Autodesk Inventor part; units mm, degrees
ref_plane "YZ Plane" through (0, 0, 0) normal (1, 0, 0) x (0, 1, 0)
ref_plane "XZ Plane" through (0, 0, 0) normal (0, 1, 0) x (-1, 0, 0)
ref_plane "XY Plane" through (0, 0, 0) normal (0, 0, 1) x (1, 0, 0)
sketch "Sketch1" plane through (0, 0, 0) normal (0, 0, 1) x (1, 0, 0)
  circle A0 centre (0, 0) radius 2 construction
  circle A1 centre (0, 0) radius 6.5 construction
  line L0 (0, 0) -> (38, 0) construction
  arc A2 (-6.8763, 10.4387) -> (-6.8763, -10.4387) centre (0, 0) ccw
  circle A3 centre (0, 0) radius 6.5
  line L1 (38, 0) -> (38, -40)
  line L2 (38, 0) -> (38, 40)
  line L3 (38, 40) -> (-6.8763, 10.4387)
  line L4 (38, -40) -> (-6.8763, -10.4387)
  point P0 (0, 0)
  dimension "d0" = 38
  dimension "d1" = 25
  dimension "d2" = 13
  dimension "d3" = 40
  dimension "d4" = 40
extrude "Extrusion1" add sketch "Sketch1" against normal blind 6
sketch "Sketch2" plane through (0, 0, -6) normal (0, 0, -1) x (-1, 0, 0)
  circle A0 centre (-13, -12.5) radius 1.5
  circle A1 centre (-13, 12.5) radius 1.5
  point P0 (0, 0)
extrude "Extrusion2" cut sketch "Sketch2" against normal blind 6
sketch "Sketch3" plane through (0, 0, -6) normal (0, 0, -1) x (-1, 0, 0)
  line L0 (-38, 40) -> (-38, -40)
  line L1 (-38, 40) -> (-38, -40) construction
  line L2 (-38, 0) -> (-63, 0) construction
  line L3 (-50, 0) -> (-50, -17)
  line L4 (-50, 0) -> (-50, 17)
  line L5 (-50, -17) -> (-38, -17)
  line L6 (-50, 17) -> (-38, 17)
  line L7 (-47.1, -14) -> (-47.1, 0)
  line L8 (-47.1, 14) -> (-47.1, 0)
  line L9 (-47.1, -14) -> (-44, -14)
  line L10 (-44, -14) -> (-44, 0)
  line L11 (-47.1, 14) -> (-44, 14)
  line L12 (-44, 14) -> (-44, 0)
  line L13 (-38, -17) -> (-38, 17)
  point P0 (0, 0)
  dimension "d9" = 25
  dimension "d10" = 17
  dimension "d11" = 12
  dimension "d12" = 14
  dimension "d13" = 2.9
  dimension "d14" = 6
extrude "Extrusion3" add sketch "Sketch3" against normal blind 6
properties part number "Mecanum wheel support"
CAD build for the part. Positions are in the model's coordinates, mm. A direction names the side the tool comes from. Round coordinates to 2 decimals unless told otherwise and drop trailing zeros. Write each loop counter-clockwise with the first axis right and the second up, starting at its lowest first coordinate (ties: lowest second). Pieces come first, ordered by that corner, then holes. Notation, with made-up numbers: M 45,19.5 L 92,19.5 A15 cw 92,34.5 Z; hole C 8.25,17 d5. An arc over 180 degrees is marked long. Put each result on its own line as item: value. Start each with the question number.
1) Pin check, flat tips, straight feed: pin 1 Ø1.5 at (x, z) = (38.5, -2) entering from -Y; pin 2 Ø1.6 at (x, z) = (45.5, -3.5) entering from -Y; pin 3 Ø1.8 at (y, z) = (27.5, -2) entering from +X; pin 4 Ø3.5 at (x, y) = (13, 12.5) entering from -Z. Stop position of each tip, or through.
2) Saw through at C-C, the plane x = 0. Write the cut outline in (y, z).
3) Saw through at A-A, the plane y = 0. Write the cut outline in (x, z), and give its area (3 significant figures).
4) Drill centre lines: probe 1 along Y at (x, z) = (13, -4.7); probe 2 along Y at (x, z) = (12, -5.05); probe 3 along X at (y, z) = (-2, -0.95). Where is each one in solid material? Low to high. Write a range as [from, to].
5) Saw through at B-B, the plane z = -2.8. Write the cut outline in (x, y), and give its area (3 significant figures).
6) Pull direction X, two halves, no side cores. Call faces 1 (the flat face through (47.1, 0, -3)), 2 (the flat face through (38, -29, -3)), 3 (the flat face through (44, -17, -3)): pulls with the +X half, pulls with the -X half, needs draft (parallel to the pull), parting line crosses it, or undercut.
7) Saw through at D-D, the plane x = 13. Write the cut outline in (y, z), and give its area (3 significant figures).
8) 3-axis set-ups, long thin cutter, end or side, ignore diameter. For faces 4 (the flat face through (44, 17, -3)), 5 (the cylindrical face through (-12.5, 0.2, -3)), 6 (the flat face through (44, 0, -3)): which of +Z, -Z, +X, -X, +Y, -Y reach the whole face in a straight line?
Resolved:
1. pin 1: y = -40
1. pin 2: y = -17
1. pin 3: x = 38
1. pin 4: z = -6
2. outline: M -14.97,-6 L -6.5,-6 L -6.5,0 L -14.97,0 Z; M 6.5,-6 L 14.97,-6 L 14.97,0 L 6.5,0 Z
3. outline: M -12.5,-6 L -6.5,-6 L -6.5,0 L -12.5,0 Z; M 6.5,-6 L 44,-6 L 44,0 L 6.5,0 Z; M 47.1,-6 L 50,-6 L 50,0 L 47.1,0 Z
3. area: 278 mm²
4. probe 1: [-23.53, -14], [-11, 11], [14, 23.53]
4. probe 2: [-22.87, -13.62], [-11.38, 11.38], [13.62, 22.87]
4. probe 3: [-12.34, -6.18], [6.18, 44], [47.1, 50]
5. outline: M -6.88,-10.44 L 38,-40 L 38,-17 L 50,-17 L 50,17 L 38,17 L 38,40 L -6.88,10.44 A12.5 ccw Z; hole C 0,0 d13; hole C 13,-12.5 d3; hole C 13,12.5 d3; hole M 44,-14 L 47.1,-14 L 47.1,14 L 44,14 Z
5. area: 2,520 mm²
6. face 1: undercut
6. face 2: pulls with the +X half
6. face 3: needs draft
7. outline: M -23.53,-6 L -14,-6 L -14,0 L -23.53,0 Z; M -11,-6 L 11,-6 L 11,0 L -11,0 Z; M 14,-6 L 23.53,-6 L 23.53,0 L 14,0 Z
7. area: 246 mm²
8. face 4: +Z, -Z, +X, +Y
8. face 5: +Z, -Z, -X
8. face 6: +Z, -Z
